```python
from build123d import *

# Parameters (mm, degrees)
EXTRUDE_1_DEPTH     = 55
SKETCH_3_W          = 47
SKETCH_3_H          = 3
EXTRUDE_2_DEPTH     = 3
SKETCH_4_W          = 45
SKETCH_4_H          = 3
EXTRUDE_3_DEPTH     = 6
SKETCH_6_R          = 1.65
CUT_EXTRUDE_1_DEPTH = 6
SKETCH_7_W          = 45
SKETCH_7_H          = 3
EXTRUDE_4_DEPTH     = 6
SKETCH_8_R          = 1.65
CUT_EXTRUDE_2_DEPTH = 6


with BuildPart() as part:
    # 草图1 → 凸台-拉伸1 (new body)
    with BuildSketch(Plane(origin=(0, 0, 0), x_dir=(1, 0, 0), z_dir=(0, 1, 0))):
        Polygon((-38.5, 0), (-35.5, 0), (-35.5, 19.5), (-23.5, 19.5), (-23.5, 22.5), (-38.5, 22.5), align=None)
        Polygon((-35.5, -19.5), (-35.5, 0), (-38.5, 0), (-38.5, -22.5), (-23.5, -22.5), (-23.5, -19.5), align=None)
        Polygon((23.5, 22.5), (23.5, 19.5), (35.5, 19.5), (35.5, -19.5), (23.5, -19.5), (23.5, -22.5), (38.5, -22.5), (38.5, 22.5), align=None)
    extrude(amount=EXTRUDE_1_DEPTH)

    # 草图3 → 凸台-拉伸2 (add)
    with BuildSketch(Plane.XZ):
        with Locations((0, 21)):
            Rectangle(SKETCH_3_W, SKETCH_3_H)
        Polygon((-35.5, 19.5), (-35.5, -19.5), (-23.5, -19.5), (23.5, -19.5), (35.5, -19.5), (35.5, 19.5), (23.5, 19.5), (-23.5, 19.5), align=None)
        with Locations((0, -21)):
            Rectangle(SKETCH_3_W, SKETCH_3_H)
    extrude(amount=-EXTRUDE_2_DEPTH)

    # 草图4 → 凸台-拉伸3 (add)
    with BuildSketch(Plane(origin=(38.5, 0, 0), x_dir=(0, 0, -1), z_dir=(1, 0, 0))):
        with Locations((0, 1.5)):
            Rectangle(SKETCH_4_W, SKETCH_4_H)
    extrude(amount=EXTRUDE_3_DEPTH)

    # 草图6 → 切除-拉伸1 (cut)
    with BuildSketch(Plane(origin=(0, 3, 0), x_dir=(1, 0, 0), z_dir=(0, 1, 0))):
        with Locations((41.5, -12.5)):
            Circle(SKETCH_6_R)
        with Locations((41.5, 12.5)):
            Circle(SKETCH_6_R)
    extrude(amount=-CUT_EXTRUDE_1_DEPTH, mode=Mode.SUBTRACT)

    # 草图7 → 凸台-拉伸4 (add)
    with BuildSketch(Plane.ZY.offset(38.5)):
        with Locations((0, 1.5)):
            Rectangle(SKETCH_7_W, SKETCH_7_H)
    extrude(amount=EXTRUDE_4_DEPTH)

    # 草图8 → 切除-拉伸2 (cut)
    with BuildSketch(Plane(origin=(0, 3, 0), x_dir=(1, 0, 0), z_dir=(0, 1, 0))):
        with Locations((-41.5, 12.5)):
            Circle(SKETCH_8_R)
        with Locations((-41.5, -12.5)):
            Circle(SKETCH_8_R)
    extrude(amount=-CUT_EXTRUDE_2_DEPTH, mode=Mode.SUBTRACT)


solid = part.part
```
Can you work these out from the model? Positions are in its coordinate system, mm. A direction names the side the tool comes from. Coordinates: 2 decimals unless noted, no trailing zeros. Loops run counter-clockwise (first coordinate to the right, second up) from the corner with the lowest first, then second, coordinate; pieces in that order, holes last. Notation, with made-up numbers: (19, 63.25) - (55, 63.25) arc R9 ccw to (55, 76.25) - close; hole circle Ø3 at (50.5, 24). An arc over 180 degrees is marked (long way). Answer as CSV lines item,"result". Start each with the question number.
1) Suppose I cut it at C-C (z = -12.5). Please give me the cut outline in (x, y).
2) Which directions (+Z, -Z, +X, -X, +Y, -Y) give clear straight access to the entire face, cutting with the end or side of a thin tool? Please do faces 1 (the flat face through (-30, 29, -19.5)), 2 (the flat face through (-23.5, 29, -21)), 3 (the flat face through (41, 3, 0)).
3) Suppose I cut it at D-D (x = -29). Please give me the cut outline in (y, z), plus the area to 3 significant figures.
4) Suppose I cut it at A-A (y = 38). Please give me the cut outline in (x, z), plus the area to 3 significant figures.
5) For pin 1 (5 mm diameter, centred on x = -13, z = 8, fed in from +Y); pin 2 (2 mm diameter, centred on y = 40.5, z = -12, fed in from +X); pin 3 (13.5 mm diameter, centred on y = 25, z = 8, fed in from -X); pin 4 (2.5 mm diameter, centred on x = 41.5, z = 12.5, fed in from -Y), each with a flat end and sliding along its axis, tell me the tip position at first contact or that it passes through.
6) I need wall thicknesses on line 1 (Z direction, x = 41.5, y = 2.3); line 2 (X direction, y = 0.8, z = -12.5); line 3 (X direction, y = 48, z = 0). Which ranges of each line are inside material? Lowest first, please. Write a range as from..to.
7) Suppose I cut it at B-B (x = -41.5). Please give me the cut outline in (y, z), plus the area to 3 significant figures.
Check result:
1,outline,"(-44.5, 0) - (-43.15, 0) - (-43.15, 3) - (-44.5, 3) - close; (-39.85, 0) - (39.85, 0) - (39.85, 3) - (38.5, 3) - (38.5, 55) - (35.5, 55) - (35.5, 3) - (-35.5, 3) - (-35.5, 55) - (-38.5, 55) - (-38.5, 3) - (-39.85, 3) - close; (43.15, 0) - (44.5, 0) - (44.5, 3) - (43.15, 3) - close"
2,face 1,"+Y"
2,face 2,"+Z, -Z, +Y"
2,face 3,"+Z, -Z, +X, +Y"
3,outline,"(0, -22.5) - (55, -22.5) - (55, -19.5) - (3, -19.5) - (3, 19.5) - (55, 19.5) - (55, 22.5) - (0, 22.5) - close"
3,area,"447 mm²"
4,outline,"(-38.5, -22.5) - (-23.5, -22.5) - (-23.5, -19.5) - (-35.5, -19.5) - (-35.5, 19.5) - (-23.5, 19.5) - (-23.5, 22.5) - (-38.5, 22.5) - close; (23.5, -22.5) - (38.5, -22.5) - (38.5, 22.5) - (23.5, 22.5) - (23.5, 19.5) - (35.5, 19.5) - (35.5, -19.5) - (23.5, -19.5) - close"
4,area,"414 mm²"
5,pin 1,"stops at y = 3"
5,pin 2,"stops at x = 38.5"
5,pin 3,"stops at x = -38.5"
5,pin 4,"passes through"
6,line 1,"z = -22.5..-14.15, -10.85..10.85, 14.15..22.5"
6,line 2,"x = -44.5..-43.15, -39.85..39.85, 43.15..44.5"
6,line 3,"x = -38.5..-35.5, 35.5..38.5"
7,outline,"(0, -22.5) - (3, -22.5) - (3, -14.15) - (0, -14.15) - close; (0, -10.85) - (3, -10.85) - (3, 10.85) - (0, 10.85) - close; (0, 14.15) - (3, 14.15) - (3, 22.5) - (0, 22.5) - close"
7,area,"115 mm²"
